Autodesk Inventor part; units mm, degrees
ref_plane "YZ Plane" through (0, 0, 0) normal (1, 0, 0) x (0, 1, 0)
ref_plane "XZ Plane" through (0, 0, 0) normal (0, 1, 0) x (-1, 0, 0)
ref_plane "XY Plane" through (0, 0, 0) normal (0, 0, 1) x (1, 0, 0)
sketch "Esboço1" plane through (0, 0, 0) normal (1, 0, 0) x (0, 1, 0)
  line L0 (0, 0) -> (0, 100)
  line L1 (0, 100) -> (10, 100)
  line L2 (10, 100) -> (10, 90.4)
  line L3 (10, 90.4) -> (50.8, 90.4)
  line L4 (50.8, 90.4) -> (50.8, 65)
  line L5 (50.8, 65) -> (10, 65)
  line L6 (10, 65) -> (10, 35)
  line L7 (10, 35) -> (50.8, 35)
  line L8 (50.8, 35) -> (50.8, 9.6)
  line L9 (50.8, 9.6) -> (10, 9.6)
  line L10 (10, 9.6) -> (10, 0)
  line L11 (10, 0) -> (0, 0)
  line L12 (0, 50) -> (10, 50)
  dimension "d0" = 10
  dimension "d1" = 100
  dimension "d2" = 25.4
  dimension "d3" = 25.4
  dimension "d4" = 15
  dimension "d5" = 15
  dimension "d6" = 50.8
revolve "Revolução1" add sketch "Esboço1" angle 360 about axis through (0, 0, 0) along (0, 0, 1)
thread "Rosca1"
thread "Rosca2"
sketch "Esboço2" plane through (0, 0, 90.4) normal (0, 0, 1) x (1, 0, 0)
  circle A0 centre (0, 0) radius 10
  circle A1 centre (0, 0) radius 45.8
  circle A2 centre (0, 0) radius 50.8
  circle A3 centre (0, 0) radius 15
  line L0 (50.5533, 5) -> (-50.5533, 5)
  line L1 (-50.5533, 5) -> (-50.5533, -5)
  line L2 (-50.5533, -5) -> (50.5533, -5)
  line L3 (50.5533, -5) -> (50.5533, 5)
  line L4 (50.5533, 5) -> (-50.5533, -5) construction
  line L5 (-50.5533, 5) -> (50.5533, -5) construction
  line L6 (5, 50.5533) -> (-5, 50.5533)
  line L7 (-5, 50.5533) -> (-5, -50.5533)
  line L8 (-5, -50.5533) -> (5, -50.5533)
  line L9 (5, -50.5533) -> (5, 50.5533)
  line L10 (5, 50.5533) -> (-5, -50.5533) construction
  line L11 (-5, 50.5533) -> (5, -50.5533) construction
  point P0 (5, 45.5263)
  point P1 (5, 14.1421)
  point P2 (14.1421, 5)
  point P3 (45.5263, 5)
  point P4 (5, -14.1421)
  point P5 (5, -45.5263)
  point P6 (45.5263, -5)
  point P7 (14.1421, -5)
  point P8 (-5, 14.1421)
  point P9 (-5, 45.5263)
  point P10 (-45.5263, 5)
  point P11 (-14.1421, 5)
  point P12 (-5, -45.5263)
  point P13 (-5, -14.1421)
  point P14 (-14.1421, -5)
  point P15 (-45.5263, -5)
  dimension "d12" = 5
  dimension "d13" = 5
  dimension "d14" = 10
  dimension "d15" = 10
extrude "Extrusão1" cut sketch "Esboço2" against normal blind 4 contours A3 L9 A1 L0 | L2 A1 L9 A3 | A3 L0 A1 L7 | L7 A1 L2 A3
sketch "Esboço3" plane through (0, 0, 9.6) normal (0, 0, -1) x (-1, 0, 0)
  circle A0 centre (0, 0) radius 10
  arc A1 (45.5263, 5) -> (5, 45.5263) centre (0, 0) ccw
  line L0 (14.1421, 5) -> (45.5263, 5)
  arc A2 (14.1421, 5) -> (5, 14.1421) centre (0, 0) ccw
  line L1 (5, 45.5263) -> (5, 14.1421)
  arc A3 (5, -14.1421) -> (14.1421, -5) centre (0, 0) ccw
  line L2 (45.5263, -5) -> (14.1421, -5)
  arc A4 (5, -45.5263) -> (45.5263, -5) centre (0, 0) ccw
  line L3 (5, -14.1421) -> (5, -45.5263)
  arc A5 (-45.5263, -5) -> (-5, -45.5263) centre (0, 0) ccw
  line L4 (-14.1421, -5) -> (-45.5263, -5)
  arc A6 (-14.1421, -5) -> (-5, -14.1421) centre (0, 0) ccw
  line L5 (-5, -45.5263) -> (-5, -14.1421)
  arc A7 (-5, 14.1421) -> (-14.1421, 5) centre (0, 0) ccw
  line L6 (-45.5263, 5) -> (-14.1421, 5)
  arc A8 (-5, 45.5263) -> (-45.5263, 5) centre (0, 0) ccw
  line L7 (-5, 14.1421) -> (-5, 45.5263)
extrude "Extrusão2" cut sketch "Esboço3" against normal blind 4 contours L0 A2 L1 A1 | A3 L2 A4 L3 | L4 A6 L5 A5 | A7 L6 A8 L7
equation "\"d3\" = d2"
equation "\"d5\" = d4"
equation "\"d15\" = d14"
properties part number "Coletor - Hand"
The listing builds one solid part. Answer for the finished solid, in the listing's coordinates (mm). A direction names the side the tool comes from. Round coordinates to 2 decimals unless told otherwise and drop trailing zeros. Loops run counter-clockwise (first coordinate to the right, second up) from the corner with the lowest first, then second, coordinate; pieces in that order, holes last. Notation, with made-up numbers: M 6,74.5 L 26,74.5 A15 cw 26,96.5 Z; hole C 67,7.25 d8. An arc over 180 degrees is marked long. Return JSON: item names as keys, results as strings.
Q1. Find the intervals of material crossed by line 1 along Z through (x, y) = (-18.5, -39.5); line 2 along X through (y, z) = (21.5, 13); line 3 along Z through (x, y) = (-25.5, -43), in increasing order. Write a range as from..to.
Results list:
{"line 1": "z = 13.6..35, 65..86.4", "line 2": "x = -46.03..-40.44, -5..5, 40.44..46.03", "line 3": "z = 9.6..35, 65..90.4"}
Q2. Find section D-D, the plane z = 50.5. Determine the outline of the cut face in (x, y), plus the area to 3 significant figures.
Results list:
{"outline": "C 0,0 d20", "area": "314 mm2"}
Q3. Find section B-B, the plane x = 0. Determine the outline of the cut face in (y, z), plus the area to 3 significant figures.
Results list:
{"outline": "M -50.8,9.6 L -10,9.6 L -10,0 L 10,0 L 10,9.6 L 50.8,9.6 L 50.8,35 L 10,35 L 10,65 L 50.8,65 L 50.8,90.4 L 10,90.4 L 10,100 L -10,100 L -10,90.4 L -50.8,90.4 L -50.8,65 L -10,65 L -10,35 L -50.8,35 Z", "area": "6,150 mm2"}
Q4. Find section A-A, the plane y = 34. Determine the outline of the cut face in (x, z), plus the area to 3 significant figures.
Results list:
{"outline": "M -37.74,9.6 L -30.69,9.6 L -30.69,13.6 L -5,13.6 L -5,9.6 L 5,9.6 L 5,13.6 L 30.69,13.6 L 30.69,9.6 L 37.74,9.6 L 37.74,35 L -37.74,35 Z; M -37.74,65 L 37.74,65 L 37.74,90.4 L 30.69,90.4 L 30.69,86.4 L 5,86.4 L 5,90.4 L -5,90.4 L -5,86.4 L -30.69,86.4 L -30.69,90.4 L -37.74,90.4 Z", "area": "3,420 mm2"}
Q5. The mould has two halves that part along Y. Classify faces 3 (the face through (32.08, 32.69, 11.57)), 4 (the face through (-1, 11, 35)), 5 (the face through (-49.592, -11.012, 22.122)): released by +Y, released by -Y, zero draft, split by the parting line, or undercut.
Results list:
{"face 3": "undercut", "face 4": "zero draft", "face 5": "split by the parting line"}
Q6. Which of the six approach directions +Z, -Z, +X, -X, +Y, -Y give full straight-line access (tool end or side, diameter ignored) to faces 1 (the face through (-5, -30, 12)), 2 (the face through (20, -20, 86.4))?
Results list:
{"face 1": "-Z", "face 2": "+Z"}
Q7. Each of these flat-tipped pins is pushed along its axis until it touches: pin 1 Ø1.5 at (x, z) = (1.5, 65) entering from -Y; pin 2 Ø4.5 at (x, z) = (-26.5, 89.5) entering from -Y; pin 3 Ø3 at (x, z) = (-24.5, 89.5) entering from +Y. Where does it stop, or does it pass through?
Results list:
{"pin 1": "stops at y = -50.79", "pin 2": "stops at y = -44.64", "pin 3": "stops at y = 45.3"}
